Build history of the part. All positions in model axes, mm. Face numbers are marked on the shaded views. Coordinates: 2 decimals unless noted, no trailing zeros. Order: outer loops, then holes, each group sorted by start corner. A loop starts at its lowest first (then second) coordinate and runs counter-clockwise, first axis right, second up. Notation, with made-up numbers: (31, 5.5) - (41, 5.5) arc R21 ccw to (41, 35.5) - close; hole circle Ø1 at (17, 53). An arc over 180 degrees is marked (long way). Return JSON: item names as keys, results as strings.
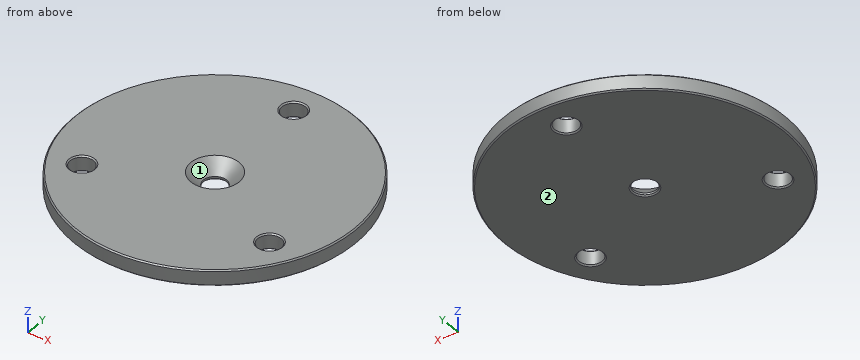
from build123d import *

# Parameters (mm, degrees)
F0_R     = 57.15
F0_R_2   = 4.7625
F1_DEPTH = 6.35
F2_SIZE  = 0.508
F3_SIZE  = 5.08


with BuildPart() as f1:
    # F0 (on Top) → F1 (new body)
    with BuildSketch(Plane.XY):
        Circle(F0_R)
        with Locations((-38.494829, -22.225)):
            Circle(F0_R_2, mode=Mode.SUBTRACT)
        with Locations((38.494829, -22.225)):
            Circle(F0_R_2, mode=Mode.SUBTRACT)
        Circle(F0_R_2, mode=Mode.SUBTRACT)
        with Locations((0, 44.45)):
            Circle(F0_R_2, mode=Mode.SUBTRACT)
    extrude(amount=F1_DEPTH)

    # F2
    f2_edges = [f1.edges().sort_by_distance(p)[0] for p in [
        (-57.15, 0, 6.35),
        (-4.7625, 44.45, 6.35),
        (-43.257329, -22.225, 6.35),
        (33.732329, -22.225, 6.35),
        (-57.15, 0, 0),
        (-4.7625, 44.45, 0),
        (33.732329, -22.225, 0),
        (-43.257329, -22.225, 0),
        (-4.7625, 0, 0),
    ]]
    chamfer(f2_edges, length=F2_SIZE)

    # F3
    f3_edges = [f1.edges().sort_by_distance(p)[0] for p in [
        (-4.7625, 0, 6.35),
    ]]
    chamfer(f3_edges, length=F3_SIZE)


solid = f1.part
1. Cut at C-C on z = 2.25. State how many separate pieces and enclosed holes the cut face has, plus the area to 3 significant figures.
Check values:
{"separate pieces": "1", "enclosed holes": "4", "area": "9,940 mm²"}
2. Probe L1, parallel to Y at x = 0, z = 0.8; L2, parallel to Y at x = 0, z = 4.7; L3, parallel to X at y = 0.5, z = 5. List the from-to ranges inside material, lowest first.
Check values:
{"L1": "-57.15 to -4.76, 4.76 to 39.69, 49.21 to 57.15", "L2": "-57.15 to -8.19, 8.19 to 39.69, 49.21 to 57.15", "L3": "-57.15 to -8.48, 8.48 to 57.15"}
3. Cut at A-A on x = 0. Give the cut face in (y, z).
Check values:
{"outline": "(-57.15, 0.51) - (-56.64, 0) - (-5.27, 0) - (-4.76, 0.51) - (-4.76, 1.27) - (-9.84, 6.35) - (-56.64, 6.35) - (-57.15, 5.84) - close; (4.76, 0.51) - (5.27, 0) - (39.18, 0) - (39.69, 0.51) - (39.69, 5.84) - (39.18, 6.35) - (9.84, 6.35) - (4.76, 1.27) - close; (49.21, 0.51) - (49.72, 0) - (56.64, 0) - (57.15, 0.51) - (57.15, 5.84) - (56.64, 6.35) - (49.72, 6.35) - (49.21, 5.84) - close"}
4. Mould opens along Y. For the marked faces 1 and 2 say: pulls with the +Y half, pulls with the -Y half, needs draft (parallel to the pull), parting line crosses it, or undercut.
Check values:
{"face 1": "undercut", "face 2": "needs draft"}
5. Drop flat-ended pins along their axis: pin 1 (3 mm diameter, centred on y = -36, z = 3, fed in from +X); pin 2 (1.5 mm diameter, centred on x = -24.5, z = 4.5, fed in from -Y); pin 3 (2 mm diameter, centred on y = -17.5, z = 2, fed in from +X); pin 4 (5.5 mm diameter, centred on x = -38.49, y = -22.22, fed in from +Z). Give the stop position or say it passes through.
Check values:
{"pin 1": "x = 45.56", "pin 2": "y = -51.98", "pin 3": "x = 54.72", "pin 4": "through"}
6. Cut at B-B on y = 0. Give the cut face in (x, z).
Check values:
{"outline": "(-57.15, 0.51) - (-56.64, 0) - (-5.27, 0) - (-4.76, 0.51) - (-4.76, 1.27) - (-9.84, 6.35) - (-56.64, 6.35) - (-57.15, 5.84) - close; (4.76, 0.51) - (5.27, 0) - (56.64, 0) - (57.15, 0.51) - (57.15, 5.84) - (56.64, 6.35) - (9.84, 6.35) - (4.76, 1.27) - close"}
